from build123d import *

# Parameters (mm, degrees)
EXTRUDE_1_DEPTH      = 5
SKETCH_4_W           = 45
SKETCH_4_H           = 30
CUT_EXTRUDE_3_DEPTH  = 5
SKETCH_5_W           = 75
SKETCH_5_H           = 160
CUT_EXTRUDE_4_DEPTH  = 5
CUT_EXTRUDE_5_REACH  = 335.054
SKETCH_6_R           = 1.5
CUT_EXTRUDE_7_REACH  = 335.054
SKETCH_7_R           = 1.6
CUT_EXTRUDE_8_REACH  = 335.054
SKETCH_8_R           = 1.5
CUT_EXTRUDE_9_REACH  = 335.054
SKETCH_9_R           = 1.5
CUT_EXTRUDE_10_REACH = 335.054
SKETCH_10_W          = 8
SKETCH_10_H          = 85


with BuildPart() as part:
    # 草图1 → 凸台-拉伸1 (new body)
    with BuildSketch(Plane(origin=(0, 0, 0), x_dir=(1, 0, 0), z_dir=(0, 1, 0))):
        with BuildLine():
            Line((10, 0), (240, 0))
            ThreePointArc((240, 0), (247.071067812, -2.928932188), (250, -10))
            Line((250, -10), (250, -210))
            ThreePointArc((250, -210), (247.071067812, -217.071067812), (240, -220))
            Line((240, -220), (10, -220))
            ThreePointArc((10, -220), (2.928932188, -217.071067812), (0, -210))
            Line((0, -210), (0, -10))
            ThreePointArc((0, -10), (2.928932188, -2.928932188), (10, 0))
        make_face()
    extrude(amount=EXTRUDE_1_DEPTH)

    # 草图4 → 切除-拉伸3 (cut)
    with BuildSketch(Plane.XZ):
        with Locations((192.5, 49.475)):
            Rectangle(SKETCH_4_W, SKETCH_4_H)
        with Locations((57.5, 49.475)):
            Rectangle(SKETCH_4_W, SKETCH_4_H)
    extrude(amount=-CUT_EXTRUDE_3_DEPTH, mode=Mode.SUBTRACT)

    # 草图5 → 切除-拉伸4 (cut)
    with BuildSketch(Plane.XZ):
        with Locations((125, 140)):
            Rectangle(SKETCH_5_W, SKETCH_5_H)
    extrude(amount=-CUT_EXTRUDE_4_DEPTH, mode=Mode.SUBTRACT)

    # 草图6 → 切除-拉伸5 (cut, up to next)
    with BuildSketch(Plane.XZ, mode=Mode.PRIVATE) as cut_extrude_5_sk1:
        with Locations(Location((72.5, 200, 0), (0, 0, 270))):
            Circle(SKETCH_6_R)
    cut_extrude_5_tool1 = extrude(cut_extrude_5_sk1.sketch, amount=-CUT_EXTRUDE_5_REACH, mode=Mode.PRIVATE) & part.part
    # 草图6 → 切除-拉伸5 (cut, up to next)
    with BuildSketch(Plane.XZ, mode=Mode.PRIVATE) as cut_extrude_5_sk2:
        with Locations(Location((177.5, 200, 0), (0, 0, 90))):
            Circle(SKETCH_6_R)
    cut_extrude_5_tool2 = extrude(cut_extrude_5_sk2.sketch, amount=-CUT_EXTRUDE_5_REACH, mode=Mode.PRIVATE) & part.part
    add(cut_extrude_5_tool1.solids().sort_by_distance((72.5, 0, 200))[0], mode=Mode.SUBTRACT)
    add(cut_extrude_5_tool2.solids().sort_by_distance((177.5, 0, 200))[0], mode=Mode.SUBTRACT)

    # 草图7 → 切除-拉伸7 (cut, up to next)
    with BuildSketch(Plane.XZ, mode=Mode.PRIVATE) as cut_extrude_7_sk1:
        with Locations(Location((17, 15, 0), (0, 0, 270))):
            Circle(SKETCH_7_R)
    cut_extrude_7_tool1 = extrude(cut_extrude_7_sk1.sketch, amount=-CUT_EXTRUDE_7_REACH, mode=Mode.PRIVATE) & part.part
    # 草图7 → 切除-拉伸7 (cut, up to next)
    with BuildSketch(Plane.XZ, mode=Mode.PRIVATE) as cut_extrude_7_sk2:
        with Locations(Location((25, 29, 0), (0, 0, 270))):
            Circle(SKETCH_7_R)
    cut_extrude_7_tool2 = extrude(cut_extrude_7_sk2.sketch, amount=-CUT_EXTRUDE_7_REACH, mode=Mode.PRIVATE) & part.part
    # 草图7 → 切除-拉伸7 (cut, up to next)
    with BuildSketch(Plane.XZ, mode=Mode.PRIVATE) as cut_extrude_7_sk3:
        with Locations(Location((25, 59, 0), (0, 0, 270))):
            Circle(SKETCH_7_R)
    cut_extrude_7_tool3 = extrude(cut_extrude_7_sk3.sketch, amount=-CUT_EXTRUDE_7_REACH, mode=Mode.PRIVATE) & part.part
    # 草图7 → 切除-拉伸7 (cut, up to next)
    with BuildSketch(Plane.XZ, mode=Mode.PRIVATE) as cut_extrude_7_sk4:
        with Locations(Location((17, 73, 0), (0, 0, 270))):
            Circle(SKETCH_7_R)
    cut_extrude_7_tool4 = extrude(cut_extrude_7_sk4.sketch, amount=-CUT_EXTRUDE_7_REACH, mode=Mode.PRIVATE) & part.part
    # 草图7 → 切除-拉伸7 (cut, up to next)
    with BuildSketch(Plane.XZ, mode=Mode.PRIVATE) as cut_extrude_7_sk5:
        with Locations(Location((233, 73, 0), (0, 0, 90))):
            Circle(SKETCH_7_R)
    cut_extrude_7_tool5 = extrude(cut_extrude_7_sk5.sketch, amount=-CUT_EXTRUDE_7_REACH, mode=Mode.PRIVATE) & part.part
    # 草图7 → 切除-拉伸7 (cut, up to next)
    with BuildSketch(Plane.XZ, mode=Mode.PRIVATE) as cut_extrude_7_sk6:
        with Locations(Location((225, 59, 0), (0, 0, 90))):
            Circle(SKETCH_7_R)
    cut_extrude_7_tool6 = extrude(cut_extrude_7_sk6.sketch, amount=-CUT_EXTRUDE_7_REACH, mode=Mode.PRIVATE) & part.part
    # 草图7 → 切除-拉伸7 (cut, up to next)
    with BuildSketch(Plane.XZ, mode=Mode.PRIVATE) as cut_extrude_7_sk7:
        with Locations(Location((225, 29, 0), (0, 0, 90))):
            Circle(SKETCH_7_R)
    cut_extrude_7_tool7 = extrude(cut_extrude_7_sk7.sketch, amount=-CUT_EXTRUDE_7_REACH, mode=Mode.PRIVATE) & part.part
    # 草图7 → 切除-拉伸7 (cut, up to next)
    with BuildSketch(Plane.XZ, mode=Mode.PRIVATE) as cut_extrude_7_sk8:
        with Locations(Location((233, 15, 0), (0, 0, 90))):
            Circle(SKETCH_7_R)
    cut_extrude_7_tool8 = extrude(cut_extrude_7_sk8.sketch, amount=-CUT_EXTRUDE_7_REACH, mode=Mode.PRIVATE) & part.part
    add(cut_extrude_7_tool1.solids().sort_by_distance((17, 0, 15))[0], mode=Mode.SUBTRACT)
    add(cut_extrude_7_tool2.solids().sort_by_distance((25, 0, 29))[0], mode=Mode.SUBTRACT)
    add(cut_extrude_7_tool3.solids().sort_by_distance((25, 0, 59))[0], mode=Mode.SUBTRACT)
    add(cut_extrude_7_tool4.solids().sort_by_distance((17, 0, 73))[0], mode=Mode.SUBTRACT)
    add(cut_extrude_7_tool5.solids().sort_by_distance((233, 0, 73))[0], mode=Mode.SUBTRACT)
    add(cut_extrude_7_tool6.solids().sort_by_distance((225, 0, 59))[0], mode=Mode.SUBTRACT)
    add(cut_extrude_7_tool7.solids().sort_by_distance((225, 0, 29))[0], mode=Mode.SUBTRACT)
    add(cut_extrude_7_tool8.solids().sort_by_distance((233, 0, 15))[0], mode=Mode.SUBTRACT)

    # 草图8 → 切除-拉伸8 (cut, up to next)
    with BuildSketch(Plane.XZ, mode=Mode.PRIVATE) as cut_extrude_8_sk1:
        with Locations(Location((235, 170, 0), (0, 0, 270))):
            Circle(SKETCH_8_R)
    cut_extrude_8_tool1 = extrude(cut_extrude_8_sk1.sketch, amount=-CUT_EXTRUDE_8_REACH, mode=Mode.PRIVATE) & part.part
    # 草图8 → 切除-拉伸8 (cut, up to next)
    with BuildSketch(Plane.XZ, mode=Mode.PRIVATE) as cut_extrude_8_sk2:
        with Locations(Location((235, 100, 0), (0, 0, 270))):
            Circle(SKETCH_8_R)
    cut_extrude_8_tool2 = extrude(cut_extrude_8_sk2.sketch, amount=-CUT_EXTRUDE_8_REACH, mode=Mode.PRIVATE) & part.part
    # 草图8 → 切除-拉伸8 (cut, up to next)
    with BuildSketch(Plane.XZ, mode=Mode.PRIVATE) as cut_extrude_8_sk3:
        with Locations(Location((15, 100, 0), (0, 0, 90))):
            Circle(SKETCH_8_R)
    cut_extrude_8_tool3 = extrude(cut_extrude_8_sk3.sketch, amount=-CUT_EXTRUDE_8_REACH, mode=Mode.PRIVATE) & part.part
    # 草图8 → 切除-拉伸8 (cut, up to next)
    with BuildSketch(Plane.XZ, mode=Mode.PRIVATE) as cut_extrude_8_sk4:
        with Locations(Location((15, 170, 0), (0, 0, 90))):
            Circle(SKETCH_8_R)
    cut_extrude_8_tool4 = extrude(cut_extrude_8_sk4.sketch, amount=-CUT_EXTRUDE_8_REACH, mode=Mode.PRIVATE) & part.part
    add(cut_extrude_8_tool1.solids().sort_by_distance((235, 0, 170))[0], mode=Mode.SUBTRACT)
    add(cut_extrude_8_tool2.solids().sort_by_distance((235, 0, 100))[0], mode=Mode.SUBTRACT)
    add(cut_extrude_8_tool3.solids().sort_by_distance((15, 0, 100))[0], mode=Mode.SUBTRACT)
    add(cut_extrude_8_tool4.solids().sort_by_distance((15, 0, 170))[0], mode=Mode.SUBTRACT)

    # 草图9 → 切除-拉伸9 (cut, up to next)
    with BuildSketch(Plane.XZ, mode=Mode.PRIVATE) as cut_extrude_9_sk1:
        with Locations(Location((77.5, 15, 0), (0, 0, 270))):
            Circle(SKETCH_9_R)
    cut_extrude_9_tool1 = extrude(cut_extrude_9_sk1.sketch, amount=-CUT_EXTRUDE_9_REACH, mode=Mode.PRIVATE) & part.part
    # 草图9 → 切除-拉伸9 (cut, up to next)
    with BuildSketch(Plane.XZ, mode=Mode.PRIVATE) as cut_extrude_9_sk2:
        with Locations(Location((10, 210, 0), (0, 0, 270))):
            Circle(SKETCH_9_R)
    cut_extrude_9_tool2 = extrude(cut_extrude_9_sk2.sketch, amount=-CUT_EXTRUDE_9_REACH, mode=Mode.PRIVATE) & part.part
    # 草图9 → 切除-拉伸9 (cut, up to next)
    with BuildSketch(Plane.XZ, mode=Mode.PRIVATE) as cut_extrude_9_sk3:
        with Locations(Location((240, 210, 0), (0, 0, 90))):
            Circle(SKETCH_9_R)
    cut_extrude_9_tool3 = extrude(cut_extrude_9_sk3.sketch, amount=-CUT_EXTRUDE_9_REACH, mode=Mode.PRIVATE) & part.part
    # 草图9 → 切除-拉伸9 (cut, up to next)
    with BuildSketch(Plane.XZ, mode=Mode.PRIVATE) as cut_extrude_9_sk4:
        with Locations(Location((172.5, 15, 0), (0, 0, 90))):
            Circle(SKETCH_9_R)
    cut_extrude_9_tool4 = extrude(cut_extrude_9_sk4.sketch, amount=-CUT_EXTRUDE_9_REACH, mode=Mode.PRIVATE) & part.part
    add(cut_extrude_9_tool1.solids().sort_by_distance((77.5, 0, 15))[0], mode=Mode.SUBTRACT)
    add(cut_extrude_9_tool2.solids().sort_by_distance((10, 0, 210))[0], mode=Mode.SUBTRACT)
    add(cut_extrude_9_tool3.solids().sort_by_distance((240, 0, 210))[0], mode=Mode.SUBTRACT)
    add(cut_extrude_9_tool4.solids().sort_by_distance((172.5, 0, 15))[0], mode=Mode.SUBTRACT)

    # 草图10 → 切除-拉伸10 (cut, up to next)
    with BuildSketch(Plane.XZ, mode=Mode.PRIVATE) as cut_extrude_10_sk1:
        with Locations((4, 42.5)):
            Rectangle(SKETCH_10_W, SKETCH_10_H)
    cut_extrude_10_tool1 = extrude(cut_extrude_10_sk1.sketch, amount=-CUT_EXTRUDE_10_REACH, mode=Mode.PRIVATE) & part.part
    # 草图10 → 切除-拉伸10 (cut, up to next)
    with BuildSketch(Plane.XZ, mode=Mode.PRIVATE) as cut_extrude_10_sk2:
        with Locations((246, 42.5)):
            Rectangle(SKETCH_10_W, SKETCH_10_H)
    cut_extrude_10_tool2 = extrude(cut_extrude_10_sk2.sketch, amount=-CUT_EXTRUDE_10_REACH, mode=Mode.PRIVATE) & part.part
    add(cut_extrude_10_tool1.solids().sort_by_distance((4, 0, 42.5))[0], mode=Mode.SUBTRACT)
    add(cut_extrude_10_tool2.solids().sort_by_distance((246, 0, 42.5))[0], mode=Mode.SUBTRACT)


solid = part.part
Can you work these out from the model? Positions are in its coordinate system, mm. A direction names the side the tool comes from. Give positions to 0.01 mm unless a question says otherwise; leave off trailing zeros. Write each loop counter-clockwise with the first axis right and the second up, starting at its lowest first coordinate (ties: lowest second). Pieces come first, ordered by that corner, then holes. Notation, with made-up numbers: (62.5, 27.25) -> (118.5, 27.25) arc R12 cw to (118.5, 41.25) -> close; hole circle Ø5 at (-20, 54). An arc over 180 degrees is marked (long way). Answer as a JSON object with one key per item and string values. Group by question number.
Item 1: I'm going to push a flat-ended pin straight in: P1, Ø2.5, axis at x = 246, y = 3, coming from the -Z side. Where does the tip first touch, or does it pass through?
Item 2: Suppose I cut it at D-D (x = 154.5). Please give me the cut outline in (y, z).
Item 3: Please list where these lines run through material, in increasing order: line 1 (X direction, y = 1.8, z = 54); line 2 (Z direction, x = 177.5, y = 1.7) (3 decimals); line 3 (Z direction, x = 202.5, y = 1.45) (3 decimals). Write a range as [from, to].
Item 4: Suppose I cut it at B-B (x = 39). Please give me the cut outline in (y, z) (3 decimals).
Item 5: Suppose I cut it at A-A (z = 82). Please give me the cut outline in (x, y), plus the area to 3 significant figures.
Item 6: For faces 1 (the face through (192, 2, 34.475)), 2 (the face through (242, 2, 42)), 3 (the face through (8, 2, 42)), which set-ups out of +Z, -Z, +X, -X, +Y, -Y let a thin tool reach every point of the face, with its end or its side?
Item 7: Suppose I cut it at C-C (y = 3.6). State how many separate pieces and enclosed holes the cut face has, plus the area to 3 significant figures.
Item 8: We'd pull the mould along X, two halves only. Please class faces 4 (the face through (192, 2, 64.475)), 5 (the face through (123, 2, 0)), 6 (the face through (0, 2, 148)), 7 (the face through (250, 2, 147)): +X half, -X half, draft (parallel to the pull), parting line (faces both ways), or undercut.
Findings:
{
 "1": {"P1": "stops at z = 85"},
 "2": {"outline": "(0, 0) -> (5, 0) -> (5, 60) -> (0, 60) -> close"},
 "3": {"line 1": "x = [8, 35], [80, 170], [215, 242]", "line 2": "z = [0, 34.475], [64.475, 198.5], [201.5, 220]", "line 3": "z = [0, 34.475], [64.475, 220]"},
 "4": {"outline": "(0, 0) -> (5, 0) -> (5, 34.475) -> (0, 34.475) -> close; (0, 64.475) -> (5, 64.475) -> (5, 220) -> (0, 220) -> close"},
 "5": {"outline": "(8, 0) -> (87.5, 0) -> (87.5, 5) -> (8, 5) -> close; (162.5, 0) -> (242, 0) -> (242, 5) -> (162.5, 5) -> close", "area": "795 mm²"},
 "6": {"face 1": "+Y, -Y", "face 2": "-Z, +X, +Y, -Y", "face 3": "-Z, -X, +Y, -Y"},
 "7": {"separate pieces": "1", "enclosed holes": "20", "area": "38,800 mm²"},
 "8": {"face 4": "undercut", "face 5": "draft", "face 6": "-X half", "face 7": "+X half"}
}
